CAD build for the part. Positions are in the model's coordinates, mm. A direction names the side the tool comes from. Give positions to 0.01 mm unless a question says otherwise; leave off trailing zeros. Write each loop counter-clockwise with the first axis right and the second up, starting at its lowest first coordinate (ties: lowest second). Pieces come first, ordered by that corner, then holes. Notation, with made-up numbers: (-33, 38.5) -> (19, 38.5) arc R34 ccw to (19, 69.5) -> close; hole circle Ø6 at (-39, -13.5). An arc over 180 degrees is marked (long way). Answer in a Markdown table with one row per item. Add a question column.
```python
from build123d import *

# Parameters (mm, degrees)
F0_W     = 1701.8
F0_H     = 1569.72
F1_DEPTH = 1422.4
F3_DEPTH = 38.1
F5_DEPTH = 317.5
F7_DEPTH = 2110.74
F6_W     = 736.6
F6_H     = 83.82
F8_DEPTH = 3215.64


with BuildPart() as f1:
    # F0 (on Front) → F1 (new body)
    with BuildSketch(Plane.XZ):
        Rectangle(F0_W, F0_H)
    extrude(amount=-F1_DEPTH)

    # F2 (on face) → F3 (cut)
    with BuildSketch(Plane.XZ):
        Polygon((728.98, -784.86), (850.9, -784.86), (850.9, -662.94), (127.4812631579, 0), (0, -116.8236655949), align=None)
        Polygon((-728.98, -784.86), (0, -116.8236655949), (-127.4812631579, 0), (-850.9, -662.94), (-850.9, -784.86), align=None)
        Polygon((0, -116.8236655949), (127.4812631579, 0), (0, 116.8236655949), (-127.4812631579, 0), align=None)
        Polygon((-127.4812631579, 0), (0, 116.8236655949), (-728.98, 784.86), (-850.9, 784.86), (-850.9, 662.94), align=None)
        Polygon((0, 116.8236655949), (127.4812631579, 0), (850.9, 662.94), (850.9, 784.86), (728.98, 784.86), align=None)
    extrude(amount=-F3_DEPTH, mode=Mode.SUBTRACT)

    # F4 (on face) → F5 (cut)
    with BuildSketch(Plane.XY.offset(784.86)):
        with BuildLine():
            ThreePointArc((0, 1291.59), (-56.5756135627, 1155.0043864373), (80.01, 1211.58))
            ThreePointArc((80.01, 1211.58), (56.5756135627, 1268.1556135627), (0, 1291.59))
        make_face()
    extrude(amount=-F5_DEPTH, mode=Mode.SUBTRACT)

    # F6 (on face) → F7 (cut)
    with BuildSketch(Plane.YZ.offset(850.9)):
        with BuildLine():
            ThreePointArc((1207.3232198715, -242.7988052368), (1191.2452582352, -119.2676443058), (1144.0826574141, -3.9674376488))
            Line((1144.0826574141, -3.9674376488), (1144.0826574141, -481.6301728248))
            ThreePointArc((1144.0826574141, -481.6301728248), (1191.2452582352, -366.3299661679), (1207.3232198715, -242.7988052368))
        make_face()
        with BuildLine():
            Line((1144.0826574141, -481.6301728248), (1144.0826574141, -3.9674376488))
            ThreePointArc((1144.0826574141, -3.9674376488), (242.1232198715, -242.7988052368), (1144.0826574141, -481.6301728248))
        make_face()
        with BuildLine():
            Line((1422.4, -486.5674376488), (1422.4, -3.9674376488))
            Line((1422.4, -3.9674376488), (1144.0826574141, -3.9674376488))
            ThreePointArc((1144.0826574141, -3.9674376488), (1191.2452582352, -119.2676443058), (1207.3232198715, -242.7988052368))
            ThreePointArc((1207.3232198715, -242.7988052368), (1191.2452582352, -366.3299661679), (1144.0826574141, -481.6301728248))
            Line((1144.0826574141, -481.6301728248), (1144.0826574141, -486.5674376488))
            Line((1144.0826574141, -486.5674376488), (1422.4, -486.5674376488))
        make_face()
    extrude(amount=-F7_DEPTH, mode=Mode.SUBTRACT)

    # F6 (on face) → F8 (cut)
    with BuildSketch(Plane.YZ.offset(850.9)):
        with Locations((1054.1, 425.45)):
            Rectangle(F6_W, F6_H)
    extrude(amount=-F8_DEPTH, mode=Mode.SUBTRACT)


solid = f1.part
```
Item 1: Slice it at A-A, the plane y = 546. List the corners of the cut face in (x, z), then the cut area to 3 significant figures.
Item 2: Slice it at B-B, the plane z = 150.5. List the corners of the cut face in (x, y).
Item 3: Slice it at D-D, the plane z = 553. List the corners of the cut face in (x, y).
Item 4: Mould opens along X. For faces 1 (the face through (850.9, 701, 338)), 2 (the face through (-369.593, 18.783, -455.518)), 3 (the face through (-12, 1422.4, 628)) say: released by +X, released by -X, zero draft, split by the parting line, or undercut.
Item 5: Drop a flat-ended pin along its axis: pin 1 Ø1.5 at (x, z) = (-45, -484.5) entering from +Y. Give the stop position or say it passes through.
Item 6: Slice it at C-C, the plane y = 846.5. List the corners of the cut face in (x, z), then the cut area to 3 significant figures.
Item 7: Probe L1, parallel to Z at x = 739.5, y = 714.5; L2, parallel to Z at x = 8, y = 707.5; L3, parallel to Y at x = 0, z = 703. List the from-to ranges inside material, lowest first. Write a range as from..to.
Item 8: Which spindle directions (+Z, -Z, +X, -X, +Y, -Y) get a long thin tool onto all of the face, cutting with end or side? Do faces 4 (the face through (-12, 1422.4, 192)), 5 (the face through (-484.13, 18.78, -326.83)), 6 (the face through (12, 685.8, 425)). Say none if no direction does.
Answer key:
| question | item | result |
|---|---|---|
| 1 | outline | (-850.9, -784.86) -> (850.9, -784.86) -> (850.9, -691.09) -> (-850.9, -691.09) -> close; (-850.9, 205.49) -> (850.9, 205.49) -> (850.9, 784.86) -> (-850.9, 784.86) -> close |
| 1 | area | 1,150,000 mm² |
| 2 | outline | (-850.9, 0) -> (-291.71, 0) -> (-291.71, 38.1) -> (-36.75, 38.1) -> (-36.75, 0) -> (36.75, 0) -> (36.75, 38.1) -> (291.71, 38.1) -> (291.71, 0) -> (850.9, 0) -> (850.9, 445.05) -> (-850.9, 445.05) -> close; (-850.9, 1004.4) -> (850.9, 1004.4) -> (850.9, 1422.4) -> (-850.9, 1422.4) -> close |
| 3 | outline | (-850.9, 0) -> (-730.93, 0) -> (-730.93, 38.1) -> (-475.97, 38.1) -> (-475.97, 0) -> (475.97, 0) -> (475.97, 38.1) -> (730.93, 38.1) -> (730.93, 0) -> (850.9, 0) -> (850.9, 1422.4) -> (-850.9, 1422.4) -> close; hole circle Ø160.02 at (0, 1211.58) |
| 4 | face 1 | released by +X |
| 4 | face 2 | undercut |
| 4 | face 3 | zero draft |
| 5 | pin 1 | stops at y = 1144.08 |
| 6 | outline | (-850.9, -784.86) -> (850.9, -784.86) -> (850.9, -709.78) -> (-850.9, -709.78) -> close; (-850.9, 224.18) -> (850.9, 224.18) -> (850.9, 383.54) -> (-850.9, 383.54) -> close; (-850.9, 467.36) -> (850.9, 467.36) -> (850.9, 784.86) -> (-850.9, 784.86) -> close |
| 6 | area | 939,000 mm² |
| 7 | L1 | z = -784.86..-725.29, 239.69..383.54, 467.36..784.86 |
| 7 | L2 | z = -784.86..-725.09, 239.49..383.54, 467.36..784.86 |
| 7 | L3 | y = 0..1131.57, 1291.59..1422.4 |
| 8 | face 4 | +Z, -Z, +X, -X, +Y |
| 8 | face 5 | -Y |
| 8 | face 6 | +X, -X, +Y |
